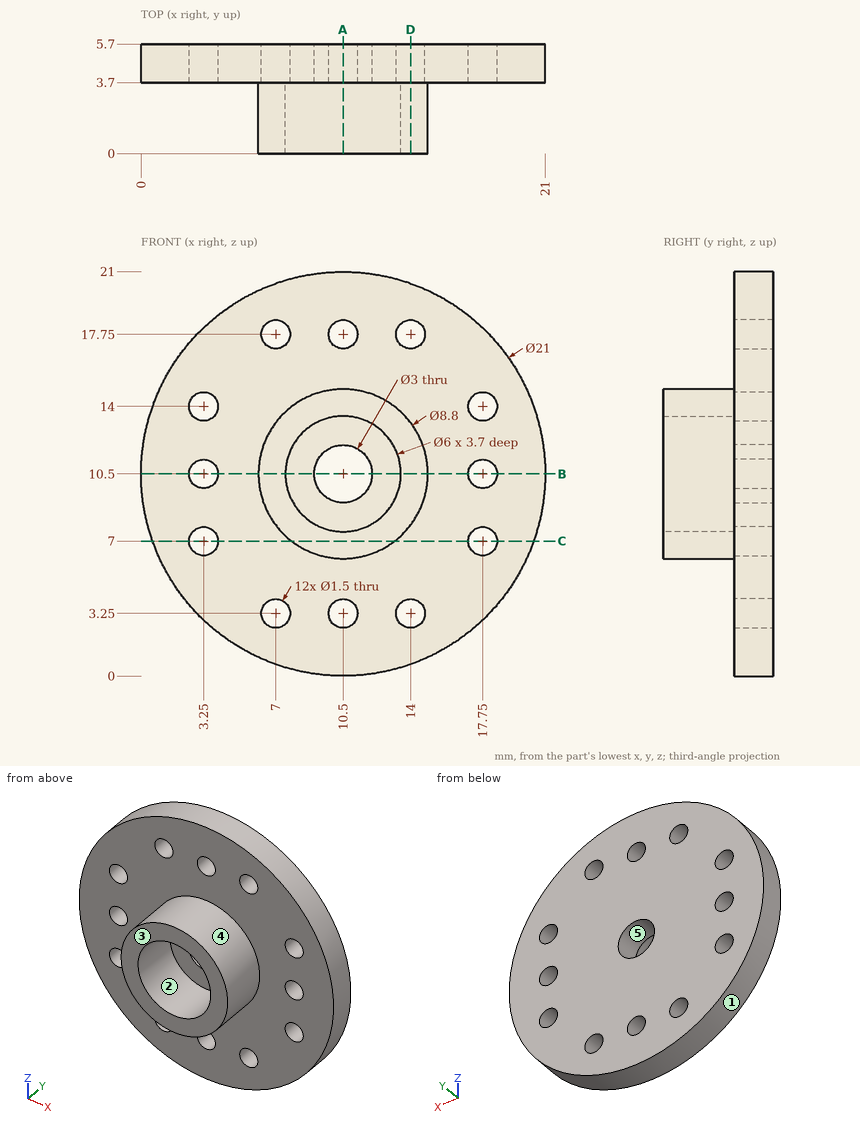
Geometry: see drawing. Coordinates: mm, zero at the bounding-box minimum. A direction names the side the tool comes from. Give positions to 0.01 mm unless a question says otherwise; leave off trailing zeros. Order: outer loops, then holes, each group sorted by start corner. A loop starts at its lowest first (then second) coordinate and runs counter-clockwise, first axis right, second up. Notation, with made-up numbers: (-11, 79.5) -> (1, 79.5) arc R5 cw to (1, 85.5) -> close; hole circle Ø1 at (-2.75, 83). An arc over 180 degrees is marked (long way). Write each question's results on one line, items separated by ' | '.
1) Cut plane D-D (x = 14). Output: boundary loops of the cut face in (y, z), and give its area (3 significant figures).
Geometry says:
outline: (0, 7.83) -> (3.7, 7.83) -> (3.7, 4) -> (5.7, 4) -> (5.7, 17) -> (3.7, 17) -> (3.7, 13.17) -> (0, 13.17) -> close; (3.7, 0.6) -> (5.7, 0.6) -> (5.7, 2.5) -> (3.7, 2.5) -> close; (3.7, 18.5) -> (5.7, 18.5) -> (5.7, 20.4) -> (3.7, 20.4) -> close | area: 53.3 mm²
2) First-contact query: pin 1 Ø2.5 at (x, z) = (10.5, 3.25) entering from +Y; pin 2 Ø2.5 at (x, z) = (3.25, 10.5) entering from -Y; pin 3 Ø1 at (y, z) = (4.5, 14.5) entering from +X; pin 4 Ø1.2 at (x, z) = (7, 3.25) entering from +Y. Flat tips, straight axial feed; report the tip coordinate or a pass-through.
Geometry says:
pin 1: stops at y = 5.7 | pin 2: stops at y = 3.7 | pin 3: stops at x = 20.4 | pin 4: passes through
3) Cut plane B-B (z = 10.5). Output: boundary loops of the cut face in (x, y).
Geometry says:
outline: (0, 3.7) -> (2.5, 3.7) -> (2.5, 5.7) -> (0, 5.7) -> close; (4, 3.7) -> (6.1, 3.7) -> (6.1, 0) -> (7.5, 0) -> (7.5, 3.7) -> (9, 3.7) -> (9, 5.7) -> (4, 5.7) -> close; (12, 3.7) -> (13.5, 3.7) -> (13.5, 0) -> (14.9, 0) -> (14.9, 3.7) -> (17, 3.7) -> (17, 5.7) -> (12, 5.7) -> close; (18.5, 3.7) -> (21, 3.7) -> (21, 5.7) -> (18.5, 5.7) -> close
4) Cut plane A-A (x = 10.5). Output: boundary loops of the cut face in (y, z).
Geometry says:
outline: (0, 6.1) -> (3.7, 6.1) -> (3.7, 4) -> (5.7, 4) -> (5.7, 9) -> (3.7, 9) -> (3.7, 7.5) -> (0, 7.5) -> close; (0, 13.5) -> (3.7, 13.5) -> (3.7, 12) -> (5.7, 12) -> (5.7, 17) -> (3.7, 17) -> (3.7, 14.9) -> (0, 14.9) -> close; (3.7, 0) -> (5.7, 0) -> (5.7, 2.5) -> (3.7, 2.5) -> close; (3.7, 18.5) -> (5.7, 18.5) -> (5.7, 21) -> (3.7, 21) -> close
5) Set-up query: the marked faces 1 and 2. Return all of +Z, -Z, +X, -X, +Y, -Y with unobstructed straight access to the full face (end or side cutting, diameter ignored); none if empty.
Geometry says:
face 1: +Y, -Y | face 2: -Y
6) Cut plane C-C (z = 7). Output: boundary loops of the cut face in (x, y), and give its area (3 significant figures).
Geometry says:
outline: (0.6, 3.7) -> (2.5, 3.7) -> (2.5, 5.7) -> (0.6, 5.7) -> close; (4, 3.7) -> (7.83, 3.7) -> (7.83, 0) -> (13.17, 0) -> (13.17, 3.7) -> (17, 3.7) -> (17, 5.7) -> (4, 5.7) -> close; (18.5, 3.7) -> (20.4, 3.7) -> (20.4, 5.7) -> (18.5, 5.7) -> close | area: 53.3 mm²
7) Line query: line 1 along X through (y, z) = (4.6, 3.25); line 2 along Z through (x, y) = (18.25, 4.5); line 3 along Y through (x, z) = (6, 19). Output: solid intervals per line, ascending.
Geometry says:
line 1: x = 2.9 to 6.25, 7.75 to 9.75, 11.25 to 13.25, 14.75 to 18.1 | line 2: z = 3.42 to 6.44, 7.56 to 9.94, 11.06 to 13.44, 14.56 to 17.58 | line 3: y = 3.7 to 5.7
8) Draft query along Z for the marked faces 3, 4 and 5. Return one class per face: released by +Z, released by -Z, zero draft, split by the parting line, or undercut.
Geometry says:
face 3: zero draft | face 4: split by the parting line | face 5: undercut
